```python
from build123d import *

# Parameters (mm, degrees)
SKETCH1_W            = 55
SKETCH1_H            = 71
BOSS_EXTRUDE1_DEPTH  = 29
SKETCH2_W            = 13
SKETCH2_H            = 15
SKETCH2_W_2          = 10
CUT_EXTRUDE1_DEPTH   = 27
CUT_EXTRUDE2_DEPTH   = 27
SKETCH4_W            = 15
SKETCH4_H            = 15
BOSS_EXTRUDE2_DEPTH  = 7
FILLET1_R            = 2
SKETCH5_R            = 2.1
CUT_EXTRUDE3_DEPTH   = 15
SKETCH6_R            = 3.75
CUT_EXTRUDE4_DEPTH   = 2
FILLET1_OF_MIRROR2_R = 2
FILLET2_R            = 2


with BuildPart() as part:
    # Sketch1 → Boss-Extrude1 (new body)
    with BuildSketch(Plane(origin=(0, 0, 0), x_dir=(1, 0, 0), z_dir=(0, 1, 0))):
        with BuildLine():
            Line((-27.5, 37.5), (27.5, 37.5))
            ThreePointArc((27.5, 37.5), (28.914213562, 36.914213562), (29.5, 35.5))
            Line((29.5, 35.5), (29.5, -35.5))
            ThreePointArc((29.5, -35.5), (28.914213562, -36.914213562), (27.5, -37.5))
            Line((27.5, -37.5), (-27.5, -37.5))
            ThreePointArc((-27.5, -37.5), (-28.914213562, -36.914213562), (-29.5, -35.5))
            Line((-29.5, -35.5), (-29.5, 35.5))
            ThreePointArc((-29.5, 35.5), (-28.914213562, 36.914213562), (-27.5, 37.5))
        make_face()
        Rectangle(SKETCH1_W, SKETCH1_H, mode=Mode.SUBTRACT)
    extrude(amount=BOSS_EXTRUDE1_DEPTH)

    # Sketch2 → Cut-Extrude1 (cut)
    with BuildSketch(Plane(origin=(0, 0, -37.5), x_dir=(-1, 0, 0), z_dir=(0, 0, -1))):
        with Locations((-13.12561668, 7.5)):
            Rectangle(SKETCH2_W, SKETCH2_H)
        with Locations((21.3, 7.5)):
            Rectangle(SKETCH2_W_2, SKETCH2_H)
    extrude(amount=-CUT_EXTRUDE1_DEPTH, mode=Mode.SUBTRACT)

    # Sketch3 → Cut-Extrude2 (cut)
    with BuildSketch(Plane(origin=(29.5, 0, 0), x_dir=(0, 0, -1), z_dir=(1, 0, 0))):
        with BuildLine():
            Line((-25.5, 22), (30.5, 22))
            ThreePointArc((30.5, 22), (31.914213562, 21.414213562), (32.5, 20))
            Line((32.5, 20), (32.5, 19))
            ThreePointArc((32.5, 19), (31.914213562, 17.585786438), (30.5, 17))
            Line((30.5, 17), (-25.5, 17))
            ThreePointArc((-25.5, 17), (-26.914213562, 17.585786438), (-27.5, 19))
            Line((-27.5, 19), (-27.5, 20))
            ThreePointArc((-27.5, 20), (-26.914213562, 21.414213562), (-25.5, 22))
        make_face()
    extrude(amount=-CUT_EXTRUDE2_DEPTH, mode=Mode.SUBTRACT)

    # Sketch4 → Boss-Extrude2 (add)
    with BuildSketch(Plane.XZ):
        with Locations((-6, 45)):
            Rectangle(SKETCH4_W, SKETCH4_H)
    boss_extrude2 = extrude(amount=-BOSS_EXTRUDE2_DEPTH)

    # Fillet1
    fillet1_edges = [part.edges().sort_by_distance(p)[0] for p in [
        (-13.5, 7, 45),
        (-6, 7, 52.5),
        (-13.5, 3.5, 52.5),
        (1.5, 7, 45),
        (1.5, 3.5, 52.5),
    ]]
    fillet(fillet1_edges, radius=FILLET1_R)

    # Sketch5 → Cut-Extrude3 (cut)
    with BuildSketch(Plane(origin=(0, 7, 0), x_dir=(1, 0, 0), z_dir=(0, 1, 0))):
        with Locations(Location((-6, -45, 0), (0, 0, 270))):  # turned: the seam where the file's is
            Circle(SKETCH5_R)
    cut_extrude3 = extrude(amount=-CUT_EXTRUDE3_DEPTH, mode=Mode.SUBTRACT)

    # Sketch6 → Cut-Extrude4 (cut)
    with BuildSketch(Plane(origin=(0, 7, 0), x_dir=(1, 0, 0), z_dir=(0, 1, 0))):
        with Locations(Location((-6, -45, 0), (0, 0, 270))):  # turned: the seam where the file's is
            Circle(SKETCH6_R)
    cut_extrude4 = extrude(amount=-CUT_EXTRUDE4_DEPTH, mode=Mode.SUBTRACT)

    # Mirror2: Boss-Extrude2, Cut-Extrude3, Cut-Extrude4 across plane
    add(boss_extrude2.mirror(Plane.XY))
    add(cut_extrude3.mirror(Plane.XY), mode=Mode.SUBTRACT)
    add(cut_extrude4.mirror(Plane.XY), mode=Mode.SUBTRACT)

    # Fillet1 of Mirror2
    fillet1_of_mirror2_edges = [part.edges().sort_by_distance(p)[0] for p in [
        (-13.5, 7, -45),
        (-6, 7, -52.5),
        (-13.5, 3.5, -52.5),
        (1.5, 7, -45),
        (1.5, 3.5, -52.5),
    ]]
    fillet(fillet1_of_mirror2_edges, radius=FILLET1_OF_MIRROR2_R)

    # Fillet2
    fillet2_edges = [part.edges().sort_by_distance(p)[0] for p in [
        (1.5, 2.5, 37.5),
        (-6, 7, 37.5),
        (-13.5, 2.5, 37.5),
        (0.914213562, 6.414213562, 37.5),
        (-12.914213562, 6.414213562, 37.5),
        (-6, 7, -37.5),
        (1.5, 2.5, -37.5),
        (-13.5, 2.5, -37.5),
        (0.914213562, 6.414213562, -37.5),
        (-12.914213562, 6.414213562, -37.5),
    ]]
    fillet(fillet2_edges, radius=FILLET2_R)


solid = part.part
```
Can you work these out from the model? Positions are in its coordinate system, mm. A direction names the side the tool comes from. Coordinates: 2 decimals unless noted, no trailing zeros. Order: outer loops, then holes, each group sorted by start corner. A loop starts at its lowest first (then second) coordinate and runs counter-clockwise, first axis right, second up.
1. I need wall thicknesses on line 1 (Z direction, x = 11.5, y = 20.75); line 2 (X direction, y = 2.4, z = -45); line 3 (X direction, y = 15.25, z = -29). Which ranges of each line are inside material? Lowest first, please.
2. I'm going to push flat-ended pins straight in: pin 1 (14.5 mm diameter, centred on x = 11.5, y = 15, fed in from -Z); pin 2 (2 mm diameter, centred on x = -6.5, y = 13.5, fed in from +Z); pin 3 (1 mm diameter, centred on y = 8.5, z = -36.5, fed in from +X). Where does each tip first touch, or does it pass through?
3. If we section it at C-C (z = -45): Please give me the cut outline in (x, y).
4. If we section it at D-D (y = 25): Please give me the cut outline in (x, z).
5. If we section it at B-B (x = 5): Please give me the cut outline in (y, z).
6. If we section it at A-A (z = -23): Please give me the cut outline in (x, y), then the cut area to 3 significant figures.
7. Thinking about a two-plate mould opening in X: for faces 1 (the face through (-5.835, 6.014, -41.254)), 2 (the face through (29, 22, -2)), 3 (the face through (28.93, 14.3, 36.9)), 4 (the face through (-13.5, 2, 45)), which applies, +X half, -X half, draft (parallel to the pull), parting line (faces both ways), or undercut?
8. For faces 5 (the face through (-26.3, 7, -37)), 6 (the face through (-27.5, 14, 0)), 7 (the face through (28.51, 17.57, 26.9)), which set-ups out of +Z, -Z, +X, -X, +Y, -Y let a thin tool reach every point of the face, with its end or its side?
Entries:
1. line 1: z = -37.5 to -35.5, 35.5 to 37.5
1. line 2: x = -13.5 to -8.1, -3.9 to 1.5
1. line 3: x = -29.5 to -27.5, 27.5 to 29.5
2. pin 1: stops at z = -37.5
2. pin 2: stops at z = 37.5
2. pin 3: stops at x = 29.44
3. outline: (-13.5, 0) - (-8.1, 0) - (-8.1, 5) - (-9.75, 5) - (-9.75, 7) - (-11.5, 7) arc R2 ccw to (-13.5, 5) - close; (-3.9, 0) - (1.5, 0) - (1.5, 5) arc R2 ccw to (-0.5, 7) - (-2.25, 7) - (-2.25, 5) - (-3.9, 5) - close
4. outline: (-29.5, -35.5) arc R2 ccw to (-27.5, -37.5) - (27.5, -37.5) arc R2 ccw to (29.5, -35.5) - (29.5, 35.5) arc R2 ccw to (27.5, 37.5) - (-27.5, 37.5) arc R2 ccw to (-29.5, 35.5) - close; hole (-27.5, -35.5) - (27.5, -35.5) - (27.5, 35.5) - (-27.5, 35.5) - close
5. outline: (0, -37.5) - (29, -37.5) - (29, -35.5) - (0, -35.5) - close; (0, 35.5) - (29, 35.5) - (29, 37.5) - (0, 37.5) - close
6. outline: (-29.5, 0) - (-27.5, 0) - (-27.5, 29) - (-29.5, 29) - close; (27.5, 0) - (29.5, 0) - (29.5, 17) - (27.5, 17) - close; (27.5, 22) - (29.5, 22) - (29.5, 29) - (27.5, 29) - close
6. area: 106 mm2
7. face 1: undercut
7. face 2: draft
7. face 3: +X half
7. face 4: -X half
8. face 5: -Z, -Y
8. face 6: +Y, -Y
8. face 7: +X
